from build123d import *

# Parameters (mm, degrees)
PAD001_DEPTH  = 5
FILLET004_R   = 7
FILLET013_R   = 2
FILLET005_R   = 1
FILLET006_R   = 1.2
SKETCH014_R   = 1.7
HOLE003_DEPTH = 25


with BuildPart() as part:
    # Sketch001 → Pad001 (new body)
    with BuildSketch(Plane.XY):
        Polygon((-9.525, 56.825), (-9.525, 47.825), (-143.075, 47.825), (-143.075, -28.775), (-119.2625, -28.775), (-119.2625, -47.825), (100.2125, -47.825), (100.2125, -28.775), (143.075, -28.775), (143.075, 47.825), (9.525, 47.825), (9.525, 56.825), (152.075, 56.825), (152.075, -56.825), (110.697365, -56.825), (94.2125, -62.825), (-113.2625, -62.825), (-129.747365, -56.825), (-152.075, -56.825), (-152.075, 56.825), align=None)
    extrude(amount=-PAD001_DEPTH)

    # Fillet004
    fillet004_edges = [part.edges().sort_by_distance(p)[0] for p in [
        (152.075, 56.825, -2.5),
        (-152.075, 56.825, -2.5),
        (-129.747365, -56.825, -2.5),
        (-113.2625, -62.825, -2.5),
        (94.2125, -62.825, -2.5),
        (110.697365, -56.825, -2.5),
    ]]
    fillet(fillet004_edges, radius=FILLET004_R)

    # Fillet013
    fillet013_edges = [part.edges().sort_by_distance(p)[0] for p in [
        (-152.075, -56.825, -2.5),
        (152.075, -56.825, -2.5),
    ]]
    fillet(fillet013_edges, radius=FILLET013_R)

    # Fillet005
    fillet005_edges = [part.edges().sort_by_distance(p)[0] for p in [
        (143.075, 47.825, -2.5),
        (-143.075, 47.825, -2.5),
        (-143.075, -28.775, -2.5),
        (-119.2625, -47.825, -2.5),
        (100.2125, -47.825, -2.5),
        (143.075, -28.775, -2.5),
    ]]
    fillet(fillet005_edges, radius=FILLET005_R)

    # Fillet006
    fillet006_edges = [part.edges().sort_by_distance(p)[0] for p in [
        (100.2125, -28.775, -2.5),
        (-119.2625, -28.775, -2.5),
    ]]
    fillet(fillet006_edges, radius=FILLET006_R)

    # Sketch014 (on Face1 of Fillet006) → Hole003 (cut)
    with BuildSketch(Plane.XY):
        with Locations((147.575, 52.325)):
            Circle(SKETCH014_R)
        with Locations((147.575, -19.05)):
            Circle(SKETCH014_R)
        with Locations((95.25, -52.325)):
            Circle(SKETCH014_R)
        with Locations((-95.25, -52.325)):
            Circle(SKETCH014_R)
        with Locations((-147.575, -19.05)):
            Circle(SKETCH014_R)
        with Locations((-147.575, 52.325)):
            Circle(SKETCH014_R)
        with Locations((-19.05, 52.325)):
            Circle(SKETCH014_R)
        with Locations((19.05, 52.325)):
            Circle(SKETCH014_R)
    extrude(amount=-HOLE003_DEPTH, mode=Mode.SUBTRACT)


solid = part.part
Could you check a few things on this model? Use its own coordinates, in mm. A direction names the side the tool comes from. Give positions to 0.01 mm unless a question says otherwise; leave off trailing zeros. Order: outer loops, then holes, each group sorted by start corner. A loop starts at its lowest first (then second) coordinate and runs counter-clockwise, first axis right, second up. Notation, with made-up numbers: (17.5, 7.25) - (29.5, 7.25) arc R16 cw to (29.5, 25.25) - close; hole circle Ø11 at (51, 7.5). An arc over 180 degrees is marked (long way). Return JSON: item names as keys, results as strings. Group by question number.
Q1. Will this pin go through, and if not, where does the flat tip stop? pin 1 Ø1.5 at (x, z) = (125, -1.5) entering from -Y (3 decimals).
Q2. Thinking about a two-plate mould opening in X: for faces 1 (the face through (143.075, 9, -2)), 2 (the face through (152.075, -2, -2)), 3 (the face through (9.525, 52, -2)), 4 (the face through (-11, -51, 0)), which applies, pulls with the +X half, pulls with the -X half, needs draft (parallel to the pull), parting line crosses it, or undercut?
Q3. Suppose I cut it at D-D, the plane z = -3.25. State how many separate pieces and enclosed holes the cut face has, and give its area (3 significant figures).
Q4. Suppose I cut it at C-C, the plane x = 3. Please give me the cut outline in (y, z) (3 decimals).
Q5. Suppose I cut it at A-A, the plane x = -38. Please give me the cut outline in (y, z) (3 decimals).
Q6. Which directions (+Z, -Z, +X, -X, +Y, -Y) give clear straight access to the entire face, cutting with the end or side of a thin tool? Please do faces 5 (the face through (-75, 47.825, -2)), 6 (the face through (-9.525, 52, -2)), 7 (the face through (150, 54.8, -2.5)).
Q7. Please list where these lines run through material, in increasing order: line 1 along Y through (x, z) = (95.25, -2.2) (3 decimals); line 2 along Y through (x, z) = (19.05, -1.5) (3 decimals); line 3 along X through (y, z) = (-38, -1) (1 decimal). Write a range as [from, to].
Q8. Suppose I cut it at B-B, the plane y = -3. Please give me the cut outline in (x, z) (3 decimals), and give its area (3 significant figures).
Resolved:
{
 "1": {"pin 1": "stops at y = -56.825"},
 "2": {"face 1": "undercut", "face 2": "pulls with the +X half", "face 3": "undercut", "face 4": "needs draft"},
 "3": {"separate pieces": "1", "enclosed holes": "8", "area": "9,540 mm2"},
 "4": {"outline": "(-62.825, -5) - (-47.825, -5) - (-47.825, 0) - (-62.825, 0) - close"},
 "5": {"outline": "(-62.825, -5) - (-47.825, -5) - (-47.825, 0) - (-62.825, 0) - close; (47.825, -5) - (56.825, -5) - (56.825, 0) - (47.825, 0) - close"},
 "6": {"face 5": "+Z, -Z", "face 6": "+Z, -Z, +Y", "face 7": "+Z, -Z, +X, +Y"},
 "7": {"line 1": "y = [-62.446, -54.025], [-50.625, -47.825], [47.825, 56.825]", "line 2": "y = [-62.825, -47.825], [47.825, 50.625], [54.025, 56.825]", "line 3": "x = [-152.1, -119.3], [100.2, 152.1]"},
 "8": {"outline": "(-152.075, -5) - (-143.075, -5) - (-143.075, 0) - (-152.075, 0) - close; (143.075, -5) - (152.075, -5) - (152.075, 0) - (143.075, 0) - close", "area": "90.0 mm2"}
}
